from build123d import *

# Parameters (mm, degrees)
SKETCH_R             = 30
PAD_DEPTH            = 4
SKETCH001_W          = 3.6
SKETCH001_H          = 3.6
POCKET_DEPTH         = 5
SKETCH002_W          = 41
SKETCH002_H          = 3.6
POCKET001_DEPTH      = 5
SKETCH003_W          = 30
SKETCH003_H          = 18
POCKET002_DEPTH      = 5
POCKET003_DEPTH      = 5
SKETCH005_R          = 0.7
POCKET004_DEPTH      = 14.701
POCKET004_DEPTH_BACK = -45.301
SKETCH006_R          = 0.7
POCKET005_DEPTH      = 9.501
POCKET005_DEPTH_BACK = -50.501
SKETCH007_W          = 21
SKETCH007_H          = 5.3
PAD001_DEPTH         = 4
SKETCH008_W          = 17.2
SKETCH008_H          = 6.2
POCKET006_DEPTH      = 5


with BuildPart() as part:
    # Sketch → Pad (new body)
    with BuildSketch(Plane.XY):
        Circle(SKETCH_R)
    extrude(amount=PAD_DEPTH)

    # Sketch001 (on Face3 of Pad) → Pocket (cut)
    with BuildSketch(Plane.XY.offset(4)):
        with Locations((-13.5, -13.5)):
            Rectangle(SKETCH001_W, SKETCH001_H)
        with Locations((13.5, -13.5)):
            Rectangle(SKETCH001_W, SKETCH001_H)
    extrude(amount=-POCKET_DEPTH, mode=Mode.SUBTRACT)

    # Sketch002 (on Face3 of Pocket) → Pocket001 (cut)
    with BuildSketch(Plane.XY.offset(4)):
        with Locations((0, 13.5)):
            Rectangle(SKETCH002_W, SKETCH002_H)
    extrude(amount=-POCKET001_DEPTH, mode=Mode.SUBTRACT)

    # Sketch003 (on Face3 of Pocket001) → Pocket002 (cut)
    with BuildSketch(Plane.XY.offset(4)):
        with Locations((0, 24.3)):
            Rectangle(SKETCH003_W, SKETCH003_H)
    extrude(amount=-POCKET002_DEPTH, mode=Mode.SUBTRACT)

    # Sketch004 (on Face3 of Pocket002) → Pocket003 (cut)
    with BuildSketch(Plane.XY.offset(4)):
        with BuildLine():
            Line((-25, 9), (25, 9))
            ThreePointArc((25, -9), (27.170645, 0), (25, 9))
            Line((-25, -9), (25, -9))
            ThreePointArc((-25, 9), (-26.90179, 0), (-25, -9))
        make_face()
        with BuildLine():
            Line((-19, -18), (19, -18))
            ThreePointArc((-19, -18), (0, -26.556025), (19, -18))
        make_face()
    extrude(amount=-POCKET003_DEPTH, mode=Mode.SUBTRACT)

    # Sketch005 (on Face12 of Pocket003) → Pocket004 (cut, two sides)
    with BuildSketch(Plane.YZ.offset(-15.3)) as pocket004_sk:
        with Locations((-13.5, 2)):
            Circle(SKETCH005_R)
    extrude(amount=-POCKET004_DEPTH, mode=Mode.SUBTRACT)
    extrude(pocket004_sk.sketch, amount=-POCKET004_DEPTH_BACK, mode=Mode.SUBTRACT)

    # Sketch006 (on Face6 of Pocket004) → Pocket005 (cut, two sides)
    with BuildSketch(Plane.YZ.offset(-20.5)) as pocket005_sk:
        with Locations((13.5, 2)):
            Circle(SKETCH006_R)
    extrude(amount=-POCKET005_DEPTH, mode=Mode.SUBTRACT)
    extrude(pocket005_sk.sketch, amount=-POCKET005_DEPTH_BACK, mode=Mode.SUBTRACT)

    # Sketch007 (on Face24 of Pocket005) → Pad001 (join)
    with BuildSketch(Plane.XY.offset(4)):
        with Locations((0, 6.35)):
            Rectangle(SKETCH007_W, SKETCH007_H)
    extrude(amount=-PAD001_DEPTH)

    # Sketch008 (on Face26 of Pad001) → Pocket006 (cut)
    with BuildSketch(Plane.XY.offset(4)):
        with Locations((0, 8.6)):
            Rectangle(SKETCH008_W, SKETCH008_H)
    extrude(amount=-POCKET006_DEPTH, mode=Mode.SUBTRACT)


solid = part.part
Build history of the part. All positions in model axes, mm. A direction names the side the tool comes from. Round coordinates to 2 decimals unless told otherwise and drop trailing zeros. Write each loop counter-clockwise with the first axis right and the second up, starting at its lowest first coordinate (ties: lowest second). Pieces come first, ordered by that corner, then holes. Notation, with made-up numbers: (69.5, 69) -> (110.5, 69) arc R24 ccw to (110.5, 94) -> close; hole circle Ø10 at (67.5, 18). An arc over 180 degrees is marked (long way). Write item = value, one per line.
(1) Two-plate mould, pull along Y, no slides. Class faces 1 (the face through (0, -9, 2)), 2 (the face through (-1.1, -29.98, 1.97)), 3 (the face through (8.6, 9, 2)): pulls with the +Y half, pulls with the -Y half, needs draft (parallel to the pull), parting line crosses it, or undercut.
Answer:
face_1 = undercut
face_2 = parting line crosses it
face_3 = needs draft
(2) Band-saw the part on B-B (x = 3). Give the cut face in (y, z), then the cut area to 3 significant figures.
Answer:
outline = (-29.85, 0) -> (-26.38, 0) -> (-26.38, 4) -> (-29.85, 4) -> close; (-18, 0) -> (-9, 0) -> (-9, 4) -> (-18, 4) -> close; (3.7, 0) -> (5.5, 0) -> (5.5, 4) -> (3.7, 4) -> close; hole circle Ø1.4 at (-13.5, 2)
area = 55.5 mm2
(3) Tool access for faces 4 (the face through (-2, -10, 4)), 5 (the face through (18, 15.3, 2)), 6 (the face through (15, 21, 2)): list every direction of +Z, -Z, +X, -X, +Y, -Y with a clear straight run to the whole face (end or side of a thin tool).
Answer:
face_4 = +Z, +X, -X, +Y, -Y
face_5 = +Z, -Z
face_6 = +Z, -Z, +Y
(4) Band-saw the part on A-A (y = 0). Give the cut face in (x, z).
Answer:
outline = (-30, 0) -> (-26.9, 0) -> (-26.9, 4) -> (-30, 4) -> close; (27.17, 0) -> (30, 0) -> (30, 4) -> (27.17, 4) -> close
(5) Band-saw the part on D-D (y = -13.5). Give the cut face in (x, z), then the cut area to 3 significant figures.
Answer:
outline = (-26.79, 0) -> (-15.3, 0) -> (-15.3, 1.3) -> (-26.79, 1.3) -> close; (-26.79, 2.7) -> (-15.3, 2.7) -> (-15.3, 4) -> (-26.79, 4) -> close; (-11.7, 0) -> (11.7, 0) -> (11.7, 1.3) -> (-11.7, 1.3) -> close; (-11.7, 2.7) -> (11.7, 2.7) -> (11.7, 4) -> (-11.7, 4) -> close; (15.3, 0) -> (26.79, 0) -> (26.79, 1.3) -> (15.3, 1.3) -> close; (15.3, 2.7) -> (26.79, 2.7) -> (26.79, 4) -> (15.3, 4) -> close
area = 121 mm2
(6) Band-saw the part on C-C (x = -23). Give the cut face in (y, z).
Answer:
outline = (-19.26, 0) -> (-9, 0) -> (-9, 4) -> (-19.26, 4) -> close; (9, 0) -> (19.26, 0) -> (19.26, 4) -> (9, 4) -> close; hole circle Ø1.4 at (-13.5, 2); hole circle Ø1.4 at (13.5, 2)
(7) Flat gauge pins, fed straight in: pin 1 (1.1 mm diameter, centred on y = -13.5, z = 1.5, fed in from +X); pin 2 (1.5 mm diameter, centred on y = -3, z = 1, fed in from -X); pin 3 (1.6 mm diameter, centred on y = -13.5, z = 2, fed in from +X). Where does each tip first touch, or does it go through?
Answer:
pin_1 = 27.06
pin_2 = -29.92
pin_3 = 27.18
(8) Probe L1, parallel to Z at x = -24.5, y = 13.5; L2, parallel to Y at x = 1, z = 1.7; L3, parallel to Y at x = -19.75, z = 2. List the from-to ranges inside material, lowest first.
Answer:
L1 = 0 to 1.3, 2.7 to 4
L2 = -29.98 to -26.54, -18 to -14.13, -12.87 to -9, 3.7 to 5.5
L3 = -22.58 to -14.2, -12.8 to -9, 9 to 11.7, 15.3 to 22.58
